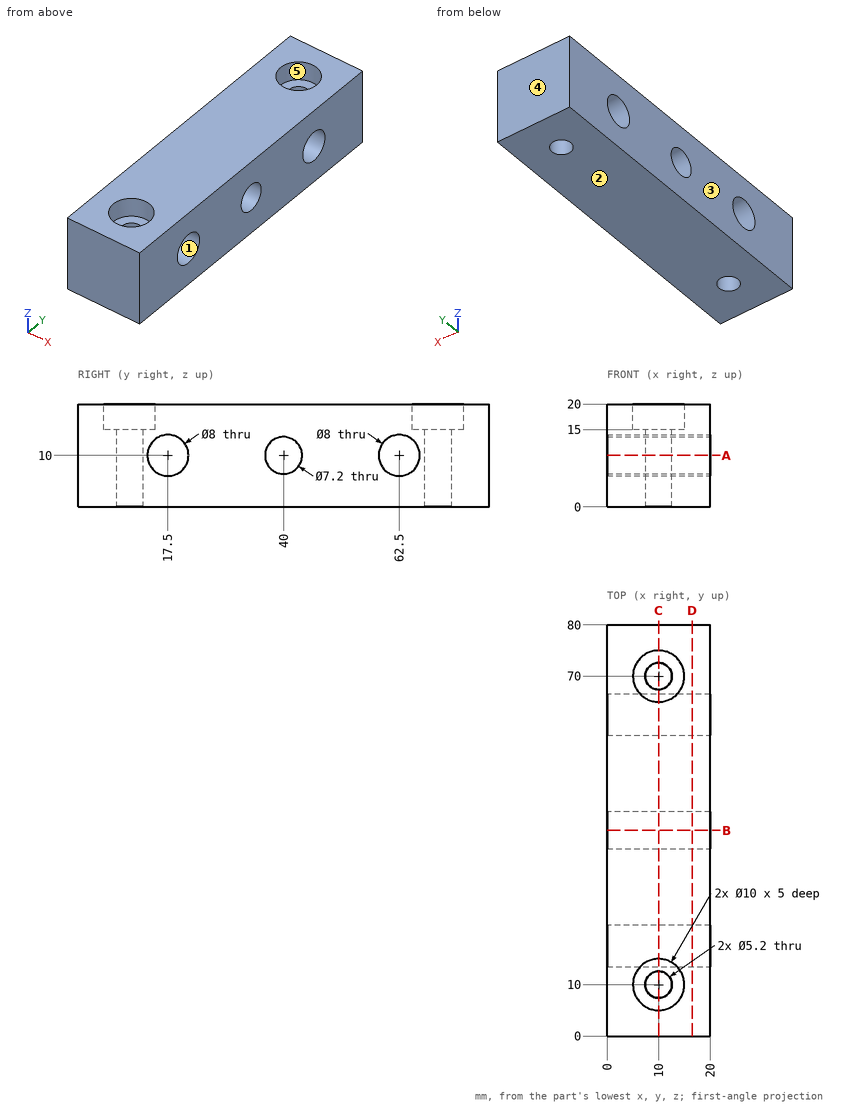
Input: dimensioned drawing with shaded views. Units: mm. Origin: part minimum x, y, z. A direction names the side the tool comes from. Give positions to 0.01 mm unless a question says otherwise; leave off trailing zeros. Write each loop counter-clockwise with the first axis right and the second up, starting at its lowest first coordinate (ties: lowest second). Pieces come first, ordered by that corner, then holes. Notation, with made-up numbers: (89.5, 73) -> (105.5, 73) arc R23 cw to (105.5, 94) -> close; hole circle Ø6 at (33.25, 10). An arc over 180 degrees is marked (long way). Return JSON: item names as keys, results as strings. Group by question number.
1. Access query for the marked faces 4 and 5. Directions: +Z, -Z, +X, -X, +Y, -Y. A direction counts if a zero-diameter tool reaches every point of the face in a straight line with its end or side. Return the directions, or none.
2. Section A-A, the plane z = 10. Output: boundary loops of the cut face in (x, y), then the cut area to 3 significant figures.
3. Section D-D, the plane x = 16.5. Output: boundary loops of the cut face in (y, z).
4. Pin query (flat end, axial travel): pin 1 Ø8 at (y, z) = (44.5, 16) entering from -X; pin 2 Ø6 at (x, y) = (10, 10) entering from +Z; pin 3 Ø4 at (x, y) = (10, 70) entering from +Z. Return the tip coordinate at first contact, or that it passes through.
5. Section C-C, the plane x = 10. Output: boundary loops of the cut face in (y, z), then the cut area to 3 significant figures.
6. Material intervals for line 1 (Y direction, x = 19, z = 10.25); line 2 (Z direction, x = 5.5, y = 62.5); line 3 (Y direction, x = 11, z = 13), sorted ascending. Write a range as from..to.
7. Mould query, pull axis Z, two halves, no side actions, for the marked faces 1, 2 and 3. Classes: +Z half, -Z half, draft (parallel to the pull), parting line (faces both ways), or undercut.
8. Section B-B, the plane y = 40. Output: boundary loops of the cut face in (x, z).
Determined:
{
 "1": {"face 4": "+Z, -Z, +X, -X, +Y", "face 5": "+Z"},
 "2": {"outline": "(0, 0) -> (20, 0) -> (20, 13.5) -> (0, 13.5) -> close; (0, 21.5) -> (20, 21.5) -> (20, 36.4) -> (0, 36.4) -> close; (0, 43.6) -> (20, 43.6) -> (20, 58.5) -> (0, 58.5) -> close; (0, 66.5) -> (20, 66.5) -> (20, 80) -> (0, 80) -> close; hole circle Ø5.2 at (10, 10); hole circle Ø5.2 at (10, 70)", "area": "1,090 mm2"},
 "3": {"outline": "(0, 0) -> (80, 0) -> (80, 20) -> (0, 20) -> close; hole circle Ø8 at (17.5, 10); hole circle Ø7.2 at (40, 10); hole circle Ø8 at (62.5, 10)"},
 "4": {"pin 1": "stops at x = 0", "pin 2": "stops at z = 15", "pin 3": "passes through"},
 "5": {"outline": "(0, 0) -> (7.4, 0) -> (7.4, 15) -> (5, 15) -> (5, 20) -> (0, 20) -> close; (12.6, 0) -> (67.4, 0) -> (67.4, 15) -> (65, 15) -> (65, 20) -> (15, 20) -> (15, 15) -> (12.6, 15) -> close; (72.6, 0) -> (80, 0) -> (80, 20) -> (75, 20) -> (75, 15) -> (72.6, 15) -> close; hole circle Ø8 at (17.5, 10); hole circle Ø7.2 at (40, 10); hole circle Ø8 at (62.5, 10)", "area": "1,200 mm2"},
 "6": {"line 1": "y = 0..13.51, 21.49..36.41, 43.59..58.51, 66.49..80", "line 2": "z = 0..6, 14..20", "line 3": "y = 0..7.6, 12.4..14.85, 20.15..38.01, 41.99..59.85, 65.15..67.6, 72.4..80"},
 "7": {"face 1": "undercut", "face 2": "-Z half", "face 3": "draft"},
 "8": {"outline": "(0, 0) -> (20, 0) -> (20, 6.4) -> (0, 6.4) -> close; (0, 13.6) -> (20, 13.6) -> (20, 20) -> (0, 20) -> close"}
}
